Study the drawing (mm; zero at the part's minimum x, y, z) and answer. A direction names the side the tool comes from. Give positions to 0.01 mm unless a question says otherwise; leave off trailing zeros. Write each loop counter-clockwise with the first axis right and the second up, starting at its lowest first coordinate (ties: lowest second). Pieces come first, ordered by that corner, then holes. Notation, with made-up numbers: (25.25, 23) - (82.25, 23) arc R16 cw to (82.25, 27) - close; hole circle Ø2 at (23, -11.75). An arc over 180 degrees is marked (long way). Answer in a Markdown table with one row per item. Add a question column.
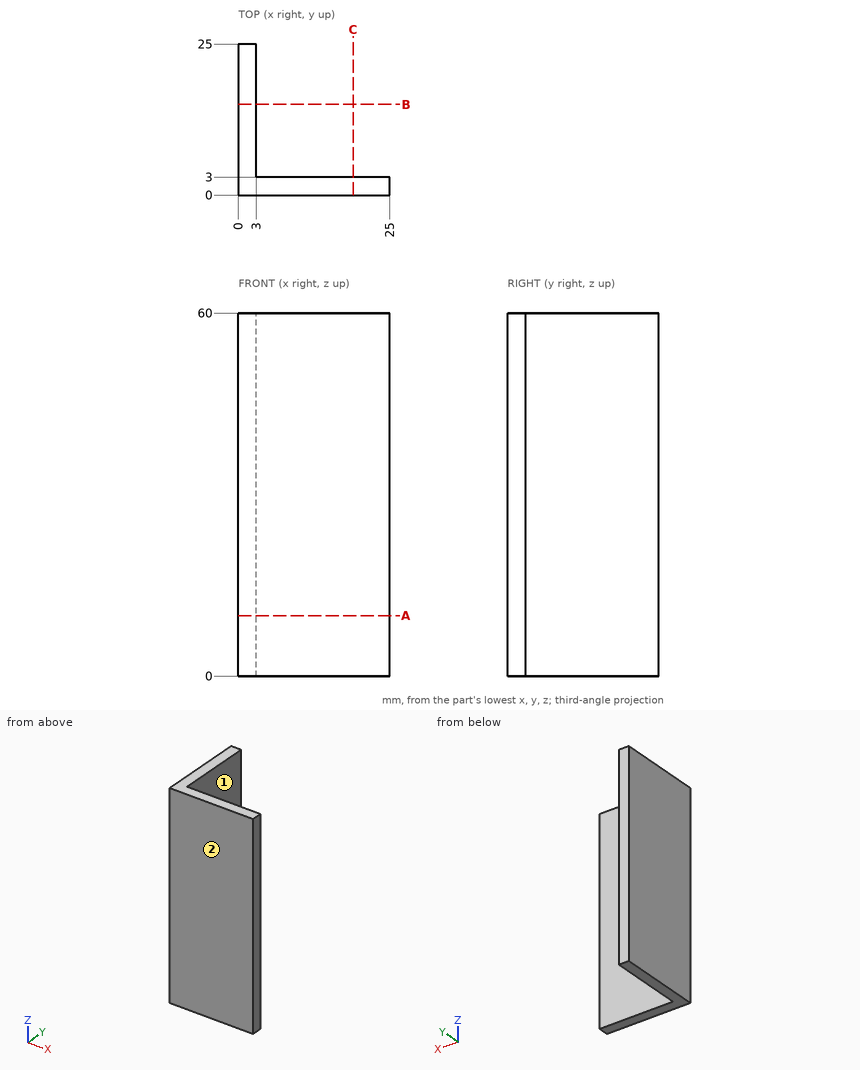
1. Section B-B (y = 15) is taken. Give the vertices of the cut face in (x, z).
2. A tool of negligible diameter and unlimited length cuts with its end or side. For the marked faces 1 and 2, from which of +Z, -Z, +X, -X, +Y, -Y can it reach the whole face along a straight path? Write none if from no direction.
3. Section A-A (z = 10) is taken. Give the vertices of the cut face in (x, y), and give its area (3 significant figures).
4. Given pin 1 Ø4 at (x, z) = (16.5, 41.5) entering from +Y; pin 2 Ø8 at (y, z) = (20.5, 32) entering from +X; pin 3 Ø10 at (x, y) = (12, 16.5) entering from +Z, each flat-ended and moving along its own axis, determine where each tip first touches the part or whether it passes through.
5. A straight line is drawn through the part: L1, parallel to Y at x = 20, z = 24.5. Find the intervals that lie inside material, in ascending order. Write a range as [from, to].
Geometry check:
| question | item | result |
|---|---|---|
| 1 | outline | (0, 0) - (3, 0) - (3, 60) - (0, 60) - close |
| 2 | face 1 | +Z, -Z, +X, +Y |
| 2 | face 2 | +Z, -Z, +X, -X, -Y |
| 3 | outline | (0, 0) - (25, 0) - (25, 3) - (3, 3) - (3, 25) - (0, 25) - close |
| 3 | area | 141 mm² |
| 4 | pin 1 | y = 3 |
| 4 | pin 2 | x = 3 |
| 4 | pin 3 | through |
| 5 | L1 | [0, 3] |
